```python
from build123d import *

# Parameters (mm, degrees)
F0_W     = 898.525
F0_H     = 317.5
F1_DEPTH = 19.05
F2_W     = 9.525
F2_H     = 9.525
F3_DEPTH = 898.526
F4_W     = 19.05
F4_H     = 19.05
F5_DEPTH = 9.525
F6_W     = 19.05
F6_H     = 19.05
F7_DEPTH = 6.35


with BuildPart() as f1:
    # F0 (on Top) → F1 (new body)
    with BuildSketch(Plane.XY):
        Rectangle(F0_W, F0_H)
    extrude(amount=F1_DEPTH)

    # F2 (on face) → F3 (cut, through all)
    with BuildSketch(Plane.YZ.offset(449.2625)):
        with Locations((153.9875, 4.7625)):
            Rectangle(F2_W, F2_H)
    extrude(amount=-F3_DEPTH, mode=Mode.SUBTRACT)

    # F4 (on face) → F5 (join)
    with BuildSketch(Plane(origin=(-449.2625, 0, 0), x_dir=(0, -1, 0), z_dir=(-1, 0, 0))):
        with Locations((149.225, 9.525)):
            Rectangle(F4_W, F4_H)
    extrude(amount=F5_DEPTH)

    # F6 (on face) → F7 (join)
    with BuildSketch(Plane.YZ.offset(449.2625)):
        with Locations((-149.225, 9.525)):
            Rectangle(F6_W, F6_H)
    extrude(amount=F7_DEPTH)


solid = f1.part
```
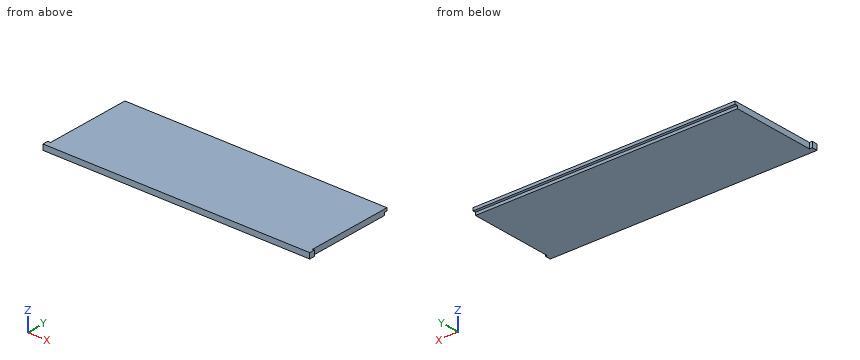
Model file for the job. Use its own axes, mm. Coordinates: 2 decimals unless noted, no trailing zeros. Order: outer loops, then holes, each group sorted by start corner. A loop starts at its lowest first (then second) coordinate and runs counter-clockwise, first axis right, second up. Notation, with made-up numbers: (-34, -3) -> (22, -3) arc R24 cw to (22, 29) -> close; hole circle Ø1 at (-18, 66.5). An arc over 180 degrees is marked (long way). Return JSON: item names as keys, results as strings.
Item 1: Slice it at A-A (z = 13.25). Write the cut outline in (x, y).
Model answer:
{"outline": "(-458.79, -158.75) -> (455.61, -158.75) -> (455.61, -139.7) -> (449.26, -139.7) -> (449.26, 158.75) -> (-449.26, 158.75) -> (-449.26, -139.7) -> (-458.79, -139.7) -> close"}
Item 2: Slice it at C-C (y = 134). Write the cut outline in (x, z).
Model answer:
{"outline": "(-449.26, 0) -> (449.26, 0) -> (449.26, 19.05) -> (-449.26, 19.05) -> close"}
Item 3: Pin check, flat tips, straight feed: P1, Ø5.5, axis at y = 21.5, z = 8, coming from the -X side; P2, Ø10.5, axis at x = 214, y = 156.5, coming from the -Z side (3 decimals); P3, Ø6, axis at y = 27, z = 14, coming from the +X side. Stop position of each tip, or through.
Model answer:
{"P1": "stops at x = -449.26", "P2": "stops at z = 9.525", "P3": "stops at x = 449.26"}
Item 4: Slice it at B-B (x = -340). Write the cut outline in (y, z) (3 decimals).
Model answer:
{"outline": "(-158.75, 0) -> (149.225, 0) -> (149.225, 9.525) -> (158.75, 9.525) -> (158.75, 19.05) -> (-158.75, 19.05) -> close"}
Item 5: Wall check: line 1 along Y through (x, z) = (-129, 9) (3 decimals); line 2 along X through (y, z) = (6.5, 6.25). Give the ranges that are in metal, low to high. Write a range as from..to.
Model answer:
{"line 1": "y = -158.75..149.225", "line 2": "x = -449.26..449.26"}
